Model file for the job. Use its own axes, mm. Coordinates: 2 decimals unless noted, no trailing zeros. Order: outer loops, then holes, each group sorted by start corner. A loop starts at its lowest first (then second) coordinate and runs counter-clockwise, first axis right, second up. Notation, with made-up numbers: (32, -6.5) -> (76, -6.5) arc R31 cw to (76, 18.5) -> close; hole circle Ø6 at (18.5, -30). An arc over 180 degrees is marked (long way). Write item = value, one per line. Start each with the question number.
Q1. Cut at C-C, the plane z = 0. List the corners of the cut face in (x, y).
Q2. Cut at B-B, the plane x = 0. List the corners of the cut face in (y, z).
Q3. Flat gauge pins, fed straight in: pin 1 (1.5 mm diameter, centred on x = 33.5, y = 1.5, fed in from -Z); pin 2 (1.5 mm diameter, centred on x = 51.5, y = 2, fed in from +Z); pin 3 (1.5 mm diameter, centred on y = 1.5, z = 4.5, fed in from +X). Where does each tip first touch, or does it go through?
Q4. Cut at A-A, the plane y = 1.6. List the corners of the cut face in (x, z) (1 decimal).
Q5. Cut at D-D, the plane x = 26.5. List the corners of the cut face in (y, z), plus the area to 3 significant figures.
Q6. Wall check: line 1 (X direction, y = 1.8, z = 0); line 2 (X direction, y = 2.15, z = 0.25); line 3 (Z direction, x = 25, y = 2.6). Give the ranges that are in metal, low to high. Write a range as from..to.
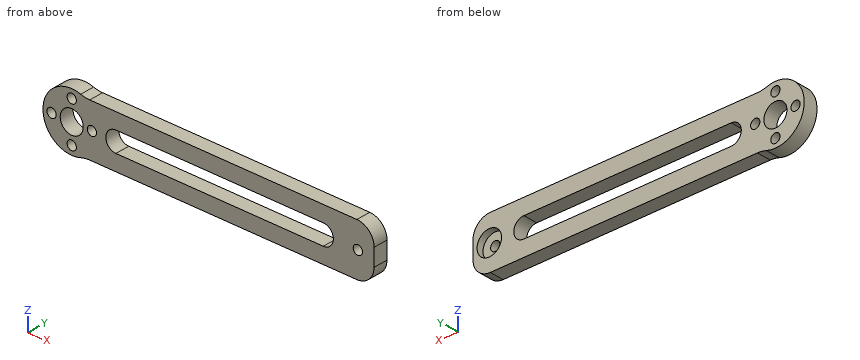
from build123d import *

# Parameters (mm, degrees)
SKETCH_1_R          = 1.6
SKETCH_1_R_2        = 9
SKETCH_1_R_3        = 4
EXTRUDE_1_DEPTH     = 5
SKETCH_2_R          = 4.25
CUT_EXTRUDE_1_DEPTH = 2.3
EXTRUDE_START       = -5
SKETCH_3_R          = 10
SKETCH_3_R_2        = 9
EXTRUDE_2_DEPTH     = 5
FILLET_1_R          = 10


with BuildPart() as part:
    # 草图1 → 凸台-拉伸1 (new body)
    # profile 1 of 2: a face of its own
    with BuildSketch(Plane(origin=(0, 0, 0), x_dir=(1, 0, 0), z_dir=(0, 1, 0))):
        with BuildLine():
            Line((99, 9), (0, 9))
            ThreePointArc((0, 9), (6.363961031, 6.363961031), (9, 0))
            ThreePointArc((9, 0), (6.363961031, -6.363961031), (0, -9))
            Line((0, -9), (99, -9))
            ThreePointArc((99, -9), (103.242640687, -7.242640687), (105, -3))
            Line((105, -3), (105, 3))
            ThreePointArc((105, 3), (103.242640687, 7.242640687), (99, 9))
        make_face()
        with BuildLine():
            ThreePointArc((15.34, -3.5), (11.84, 0), (15.34, 3.5))
            Line((15.34, 3.5), (87.34, 3.5))
            ThreePointArc((87.34, 3.5), (90.84, 0), (87.34, -3.5))
            Line((87.34, -3.5), (15.34, -3.5))
        make_face(mode=Mode.SUBTRACT)
        with Locations(Location((99.34, 0, 0), (0, 0, 270))):
            Circle(SKETCH_1_R, mode=Mode.SUBTRACT)
    # profile 2 of 2: a face of its own
    with BuildSketch(Plane(origin=(0, 0, 0), x_dir=(1, 0, 0), z_dir=(0, 1, 0))):
        Circle(SKETCH_1_R_2)
        with Locations(Location((0, -7, 0), (0, 0, 270))):
            Circle(SKETCH_1_R, mode=Mode.SUBTRACT)
        with Locations(Location((7, 0, 0), (0, 0, 270))):
            Circle(SKETCH_1_R, mode=Mode.SUBTRACT)
        with Locations(Location((0, 7, 0), (0, 0, 270))):
            Circle(SKETCH_1_R, mode=Mode.SUBTRACT)
        with Locations(Location((-7, 0, 0), (0, 0, 270))):
            Circle(SKETCH_1_R, mode=Mode.SUBTRACT)
        with Locations(Location((0, 0, 0), (0, 0, 270))):
            Circle(SKETCH_1_R_3, mode=Mode.SUBTRACT)
    extrude(amount=EXTRUDE_1_DEPTH)

    # 草图2 → 切除-拉伸1 (cut)
    with BuildSketch(Plane(origin=(0, 5, 0), x_dir=(1, 0, 0), z_dir=(0, 1, 0))):
        with Locations(Location((99.34, 0, 0), (0, 0, 270))):
            Circle(SKETCH_2_R)
    extrude(amount=-CUT_EXTRUDE_1_DEPTH, mode=Mode.SUBTRACT)

    # 草图3 → 凸台-拉伸2 (add)
    with BuildSketch(Plane(origin=(0, 5, 0), x_dir=(1, 0, 0), z_dir=(0, 1, 0)).offset(EXTRUDE_START)):
        Circle(SKETCH_3_R)
        Circle(SKETCH_3_R_2, mode=Mode.SUBTRACT)
    extrude(amount=EXTRUDE_2_DEPTH)

    # 圆角1
    fillet_1_edges = [part.edges().sort_by_distance(p)[0] for p in [
        (4.358898944, 2.5, -9),
        (4.358898944, 2.5, 9),
    ]]
    fillet(fillet_1_edges, radius=FILLET_1_R)


solid = part.part
Here are the results:
q1.outline = (-10, 0) -> (-8.6, 0) -> (-8.6, 5) -> (-10, 5) -> close; (-5.4, 0) -> (-4, 0) -> (-4, 5) -> (-5.4, 5) -> close; (4, 0) -> (5.4, 0) -> (5.4, 5) -> (4, 5) -> close; (8.6, 0) -> (11.84, 0) -> (11.84, 5) -> (8.6, 5) -> close; (90.84, 0) -> (97.74, 0) -> (97.74, 2.7) -> (95.09, 2.7) -> (95.09, 5) -> (90.84, 5) -> close; (100.94, 0) -> (105, 0) -> (105, 5) -> (103.59, 5) -> (103.59, 2.7) -> (100.94, 2.7) -> close
q2.outline = (0, -10) -> (5, -10) -> (5, -8.6) -> (0, -8.6) -> close; (0, -5.4) -> (5, -5.4) -> (5, -4) -> (0, -4) -> close; (0, 4) -> (5, 4) -> (5, 5.4) -> (0, 5.4) -> close; (0, 8.6) -> (5, 8.6) -> (5, 10) -> (0, 10) -> close
q3.pin_1 = -9
q3.pin_2 = 9
q3.pin_3 = 104.95
q4.outline = (3.1, -9.5) arc R10 cw to (6.2, -9) -> (99, -9) arc R6 ccw to (105, -3) -> (105, 3) arc R6 ccw to (99, 9) -> (6.2, 9) arc R10 cw to (3.1, 9.5) arc R10 ccw (long way) to start; hole circle Ø3.2 at (-7, 0); hole circle Ø8 at (0, 0); hole circle Ø3.2 at (0, -7); hole circle Ø3.2 at (0, 7); hole circle Ø3.2 at (7, 0); hole (15.3, -3.5) -> (87.3, -3.5) arc R3.5 ccw to (87.3, 3.5) -> (15.3, 3.5) arc R3.5 ccw to start; hole circle Ø3.2 at (99.3, 0)
q5.outline = (0, -9) -> (5, -9) -> (5, -3.5) -> (0, -3.5) -> close; (0, 3.5) -> (5, 3.5) -> (5, 9) -> (0, 9) -> close
q5.area = 55.0 mm²
q6.line_1 = -10..-8.6, -5.4..-4, 4..5.4, 8.6..11.84, 90.84..97.74, 100.94..105
q6.line_2 = -10..-8.58, -5.42..-3.99, 3.99..5.42, 8.58..11.85, 90.83..97.76, 100.92..105
q6.line_3 = -9..-3.5, 3.5..9
